Could you check a few things on this model? Use its own coordinates, in mm. A direction names the side the tool comes from. Coordinates: 2 decimals unless noted, no trailing zeros. Loops run counter-clockwise (first coordinate to the right, second up) from the corner with the lowest first, then second, coordinate; pieces in that order, holes last. Notation, with made-up numbers: (67.25, 37.5) - (114.25, 37.5) arc R18 ccw to (114.25, 52.5) - close; hole circle Ø3 at (89, -37). An arc over 180 degrees is marked (long way). One line per item, written item: value. Start each with the question number.
(1) On a 3-axis mill with a long thin cutter (end or side, diameter ignored), from which of +Z, -Z, +X, -X, +Y, -Y can I reach the whole of each face in a straight line? I mean faces 1 (the face through (-4, 0, 0)), 2 (the face through (-44.75, 4, 14)), 3 (the face through (-44.75, 4, -14)). Say none if no direction works.
(2) I'm going to push flat-ended pins straight in: P1, Ø2.5, axis at x = -42.25, z = 16.5, coming from the +Y side; P2, Ø2, axis at x = -49.5, y = 4, coming from the -Z side. Where does each tip first touch, or does it pass through?
(3) If we section it at D-D on z = 11: Write out the boundary of the cut face in (x, y), then the cut area to 3 significant figures.
(4) If we mould it in two halves opening along Z, with no side actions, what happens to faces 4 (the face through (-1, 4, -19)), 5 (the face through (-43.714, 4.056, 16.175)), 6 (the face through (-43.714, 4.056, -16.825)), 7 (the face through (44.75, 4, 0))? For each: pulls with the +Z half, pulls with the -Z half, needs draft (parallel to the pull), parting line crosses it, or undercut.
(5) If we section it at B-B on z = -16.5: Write out the boundary of the cut face in (x, y).
(6) If we section it at A-A on x = 42.25: Write out the boundary of the cut face in (y, z).
(7) If I drill on line 1 along X through (y, z) = (4, 16.5); line 2 along X through (y, z) = (1.5, 15.5); line 3 along X through (y, z) = (1, 11), over which ranges is the centre line in solid material (lowest first)? Write a range as from..to.
(8) If we section it at C-C on y = 4.25: Write out the boundary of the cut face in (x, z).
```python
from build123d import *

# Parameters (mm, degrees)
SKETCH1_W           = 89.5
SKETCH1_H           = 38
BOSS_EXTRUDE1_DEPTH = 8
SKETCH2_R           = 1.5
CUT_EXTRUDE1_DEPTH  = 50.270300385
FILLET1_R           = 1
SKETCH4_W           = 6.5
SKETCH4_H           = 20
BOSS_EXTRUDE2_DEPTH = 8


with BuildPart() as part:
    # Sketch1 → Boss-Extrude1 (new body)
    with BuildSketch(Plane(origin=(0, 0, 0), x_dir=(1, 0, 0), z_dir=(0, 1, 0))):
        Rectangle(SKETCH1_W, SKETCH1_H)
    extrude(amount=BOSS_EXTRUDE1_DEPTH)

    # Sketch2 → Cut-Extrude1 (cut, through all)
    with BuildSketch(Plane(origin=(0, 8, 0), x_dir=(1, 0, 0), z_dir=(0, 1, 0))):
        with Locations(Location((-42.25, 16.5, 0), (0, 0, 270))):
            Circle(SKETCH2_R)
        with Locations(Location((42.25, 16.5, 0), (0, 0, 270))):
            Circle(SKETCH2_R)
        with Locations(Location((42.25, -16.5, 0), (0, 0, 270))):
            Circle(SKETCH2_R)
        with Locations(Location((-42.25, -16.5, 0), (0, 0, 270))):
            Circle(SKETCH2_R)
    extrude(amount=-CUT_EXTRUDE1_DEPTH, mode=Mode.SUBTRACT)

    # Fillet1
    fillet1_edges = [part.edges().sort_by_distance(p)[0] for p in [
        (44.75, 4, 19),
        (-44.75, 4, 19),
        (-44.75, 4, -19),
        (44.75, 4, -19),
    ]]
    fillet(fillet1_edges, radius=FILLET1_R)

    # Sketch4 → Boss-Extrude2 (add)
    with BuildSketch(Plane(origin=(0, 8, 0), x_dir=(1, 0, 0), z_dir=(0, 1, 0))):
        with Locations((-48, 0)):
            Rectangle(SKETCH4_W, SKETCH4_H)
    extrude(amount=-BOSS_EXTRUDE2_DEPTH)


solid = part.part
```
Values:
1. face 1: +Z, -Z, +X, -X, -Y
1. face 2: +Z, -X, +Y, -Y
1. face 3: -Z, -X, +Y, -Y
2. P1: passes through
2. P2: stops at z = -10
3. outline: (-44.75, 0) - (44.75, 0) - (44.75, 8) - (-44.75, 8) - close
3. area: 716 mm2
4. face 4: pulls with the -Z half
4. face 5: undercut
4. face 6: undercut
4. face 7: needs draft
5. outline: (-44.75, 0) - (-43.75, 0) - (-43.75, 8) - (-44.75, 8) - close; (-40.75, 0) - (40.75, 0) - (40.75, 8) - (-40.75, 8) - close; (43.75, 0) - (44.75, 0) - (44.75, 8) - (43.75, 8) - close
6. outline: (0, -19) - (8, -19) - (8, -18) - (0, -18) - close; (0, -15) - (8, -15) - (8, 15) - (0, 15) - close; (0, 18) - (8, 18) - (8, 19) - (0, 19) - close
7. line 1: x = -44.75..-43.75, -40.75..40.75, 43.75..44.75
7. line 2: x = -44.75..-43.37, -41.13..41.13, 43.37..44.75
7. line 3: x = -44.75..44.75
8. outline: (-51.25, -10) - (-44.75, -10) - (-44.75, -18) arc R1 ccw to (-43.75, -19) - (43.75, -19) arc R1 ccw to (44.75, -18) - (44.75, 18) arc R1 ccw to (43.75, 19) - (-43.75, 19) arc R1 ccw to (-44.75, 18) - (-44.75, 10) - (-51.25, 10) - close; hole circle Ø3 at (-42.25, -16.5); hole circle Ø3 at (-42.25, 16.5); hole circle Ø3 at (42.25, -16.5); hole circle Ø3 at (42.25, 16.5)
